from build123d import *

# Parameters (mm, degrees)
F0_W           = 130
F0_H           = 50
F1_DEPTH       = 19.05
F2_R           = 18
F3_DEPTH       = 40
F4_D           = 8.8
F4_CBORE_D     = 14.25
F4_CBORE_DEPTH = 8
F6_D           = 8.8
F6_CBORE_D     = 14.25
F6_CBORE_DEPTH = 8
F7_W           = 21.662
F7_H           = 5
F8_DEPTH       = 40
F10_DEPTH      = 25


with BuildPart() as f1:
    # F0 (on Front) → F1 (new body)
    with BuildSketch(Plane.XZ):
        with Locations((65, 25)):
            Rectangle(F0_W, F0_H)
    extrude(amount=F1_DEPTH)

    # F2 (on Front) → F3 (cut)
    with BuildSketch(Plane.XZ):
        with Locations((35, 25)):
            Circle(F2_R)
    extrude(amount=F3_DEPTH, mode=Mode.SUBTRACT)

    # F4 (through all)
    with Locations(Plane(origin=(0, 0, 0), x_dir=(1, 0, 0), z_dir=(0, 1, 0))):
        with Locations((110, -25)):
            CounterBoreHole(F4_D / 2, F4_CBORE_D / 2, F4_CBORE_DEPTH)

    # F6 (through all)
    with Locations(Plane.XY.offset(50)):
        with Locations((10, -9.525)):
            CounterBoreHole(F6_D / 2, F6_CBORE_D / 2, F6_CBORE_DEPTH)

    # F7 (on face) → F8 (cut)
    with BuildSketch(Plane(origin=(0, 0, 0), x_dir=(-1, 0, 0), z_dir=(0, 1, 0))):
        with Locations((-10.831, 25)):
            Rectangle(F7_W, F7_H)
    extrude(amount=-F8_DEPTH, mode=Mode.SUBTRACT)

    # F9 (on face) → F10 (cut)
    with BuildSketch(Plane(origin=(0, 0, 0), x_dir=(-1, 0, 0), z_dir=(0, 1, 0))):
        Polygon((-130, 19), (-130, 0), (-111, 0), align=None)
        Polygon((-130, 50), (-130, 31), (-111, 50), align=None)
    extrude(amount=-F10_DEPTH, mode=Mode.SUBTRACT)


solid = f1.part
Part model, mm, in its own coordinate system. A direction names the side the tool comes from. Coordinates: 2 decimals unless noted, no trailing zeros. Loops run counter-clockwise (first coordinate to the right, second up) from the corner with the lowest first, then second, coordinate; pieces in that order, holes last. Notation, with made-up numbers: (56, 73) -> (103, 73) arc R22 ccw to (103, 105) -> close; hole circle Ø8 at (35.5, 15.25). An arc over 180 degrees is marked (long way). Use a Markdown table: item, result. Add a question column.
Item 1: Band-saw the part on A-A on z = 33.5. Write the cut outline in (x, y) (3 decimals).
Item 2: Band-saw the part on B-B on y = -11. Write the cut outline in (x, z), plus the area to 3 significant figures.
Item 3: Band-saw the part on C-C on x = 10. Write the cut outline in (y, z) (3 decimals).
Item 4: Probe probe 1 along Z at (x, y) = (110, -2) (3 decimals); probe 2 along X at (y, z) = (-11.5, 24.5); probe 3 along X at (y, z) = (-13, 19). List the from-to ranges inside material, lowest first.
Item 5: Band-saw the part on D-D on x = 35. Write the cut outline in (y, z).
Item 6: Flat gauge pins, fed straight in: P1, Ø14, axis at x = 110, z = 25, coming from the +Y side; P2, Ø8.5, axis at x = 8.5, y = -11, coming from the +Z side. Where does each tip first touch, or does it go through?
Item 7: Pull direction X, two halves, no side cores. Call faces 1 (the cylindrical face through (5.803, -8.203, 11.093)), 2 (the flat face through (5, -9, 27.5)), 3 (the flat face through (120, -9, 9)): +X half, -X half, draft (parallel to the pull), parting line (faces both ways), or undercut.
Item 8: Which spindle directions (+Z, -Z, +X, -X, +Y, -Y) get a long thin tool onto all of the face, cutting with end or side? Do faces 4 (the cylindrical face through (13.8, -3.5, 46.1)), 5 (the cylindrical face through (114.396, -13.602, 24.807)), 6 (the flat face through (5, -9, 22.5)), 7 (the cylindrical face through (104.35, -3.94, 29.34)). Say none if no direction does.
Geometry says:
| question | item | result |
|---|---|---|
| 1 | outline | (0, -19.05) -> (19.133, -19.05) -> (19.133, 0) -> (0, 0) -> close; (50.867, -19.05) -> (127.5, -19.05) -> (127.5, 0) -> (50.867, 0) -> close; hole circle Ø8.8 at (10, -9.525) |
| 2 | outline | (0, 0) -> (5.85, 0) -> (5.85, 22.5) -> (0, 22.5) -> close; (0, 27.5) -> (5.85, 27.5) -> (5.85, 42) -> (3.03, 42) -> (3.03, 50) -> (0, 50) -> close; (14.15, 0) -> (111, 0) -> (130, 19) -> (130, 31) -> (111, 50) -> (16.97, 50) -> (16.97, 42) -> (14.15, 42) -> (14.15, 27.5) -> (17.17, 27.5) arc R18 cw (long way) to (17.17, 22.5) -> (14.15, 22.5) -> close; hole circle Ø8.8 at (110, 25) |
| 2 | area | 4,560 mm² |
| 3 | outline | (-19.05, 0) -> (-13.925, 0) -> (-13.925, 22.5) -> (-19.05, 22.5) -> close; (-19.05, 27.5) -> (-13.925, 27.5) -> (-13.925, 42) -> (-16.65, 42) -> (-16.65, 50) -> (-19.05, 50) -> close; (-5.125, 0) -> (0, 0) -> (0, 22.5) -> (-5.125, 22.5) -> close; (-5.125, 27.5) -> (0, 27.5) -> (0, 50) -> (-2.4, 50) -> (-2.4, 42) -> (-5.125, 42) -> close |
| 4 | probe 1 | 0 to 17.875, 32.125 to 50 |
| 4 | probe 2 | 52.99 to 105.63, 114.37 to 130 |
| 4 | probe 3 | 0 to 7.3, 12.7 to 18.03, 51.97 to 130 |
| 5 | outline | (-19.05, 0) -> (0, 0) -> (0, 7) -> (-19.05, 7) -> close; (-19.05, 43) -> (0, 43) -> (0, 50) -> (-19.05, 50) -> close |
| 6 | P1 | y = -8 |
| 6 | P2 | z = 42 |
| 7 | face 1 | undercut |
| 7 | face 2 | draft |
| 7 | face 3 | +X half |
| 8 | face 4 | +Z |
| 8 | face 5 | +Y, -Y |
| 8 | face 6 | -X, +Y, -Y |
| 8 | face 7 | +Y |
